The model under review builds one solid part; all positions refer to its coordinate system, in mm. A direction names the side the tool comes from. Coordinates: 2 decimals unless noted, no trailing zeros. Write each loop counter-clockwise with the first axis right and the second up, starting at its lowest first coordinate (ties: lowest second). Pieces come first, ordered by that corner, then holes.
```python
from build123d import *

# Parameters (mm, degrees)
SKETCH1_R               = 9.525
BOSS_EXTRUDE1_DEPTH     = 9.525
SKETCH2_R               = 3.175
BOSS_EXTRUDE2_DEPTH     = 12.7
SKETCH3_R               = 4.7625
CUT_EXTRUDE1_DEPTH      = 10.525
CUT_EXTRUDE1_DEPTH_BACK = 10.525


with BuildPart() as part:
    # Sketch1 → Boss-Extrude1 (new body, symmetric)
    with BuildSketch(Plane.XY):
        Circle(SKETCH1_R)
    extrude(amount=BOSS_EXTRUDE1_DEPTH, both=True)

    # Sketch2 → Boss-Extrude2 (add, symmetric)
    with BuildSketch(Plane.XY):
        Circle(SKETCH2_R)
    extrude(amount=BOSS_EXTRUDE2_DEPTH, both=True)

    # Sketch3 → Cut-Extrude1 (cut, two sides)
    with BuildSketch(Plane(origin=(0, 0, 0), x_dir=(0, 0, -1), z_dir=(1, 0, 0))) as cut_extrude1_sk:
        Circle(SKETCH3_R)
    extrude(amount=CUT_EXTRUDE1_DEPTH, mode=Mode.SUBTRACT)
    extrude(cut_extrude1_sk.sketch, amount=-CUT_EXTRUDE1_DEPTH_BACK, mode=Mode.SUBTRACT)


solid = part.part
```
Item 1: Take a section at D-D, the plane y = 2.5. Write out the cut boundary in (x, z) (3 decimals), plus the area to 3 significant figures.
Solved:
outline: (-9.191, -9.525) - (-1.957, -9.525) - (-1.957, -12.7) - (1.957, -12.7) - (1.957, -9.525) - (9.191, -9.525) - (9.191, -4.054) - (-9.191, -4.054) - close; (-9.191, 4.054) - (9.191, 4.054) - (9.191, 9.525) - (1.957, 9.525) - (1.957, 12.7) - (-1.957, 12.7) - (-1.957, 9.525) - (-9.191, 9.525) - close
area: 226 mm2
Item 2: Take a section at C-C, the plane z = 2.25. Write out the cut boundary in (x, y) (3 decimals).
Solved:
outline: (-8.55, -4.197) arc R9.525 ccw to (8.55, -4.197) - close; (-8.55, 4.197) - (8.55, 4.197) arc R9.525 ccw to start
Item 3: Take a section at A-A, the plane y = 0. Write out the cut boundary in (x, z) (1 decimal).
Solved:
outline: (-9.5, -9.5) - (-3.2, -9.5) - (-3.2, -12.7) - (3.2, -12.7) - (3.2, -9.5) - (9.5, -9.5) - (9.5, -4.8) - (-9.5, -4.8) - close; (-9.5, 4.8) - (9.5, 4.8) - (9.5, 9.5) - (3.2, 9.5) - (3.2, 12.7) - (-3.2, 12.7) - (-3.2, 9.5) - (-9.5, 9.5) - close
Item 4: Machinability: for faces 1 (the face through (-0.69, -3.1, 11.13)), 2 (the face through (0, 0, 12.7)), 3 (the face through (4, 0, -9.525)), which of the approach directions +Z, -Z, +X, -X, +Y, -Y give a long, thin tool a straight path to every point of the face, cutting with its end or side? Answer none if there is none.
Solved:
face 1: +Z
face 2: +Z, +X, -X, +Y, -Y
face 3: -Z
Item 5: To check wall thickness, follow line 1 along Z through (x, y) = (-2.5, 0); line 2 along Z through (x, y) = (4.75, 0) (1 decimal); line 3 along Y through (x, z) = (-5, 0). State the ranges of each line that lie inside material, in increasing order.
Solved:
line 1: z = -12.7 to -4.76, 4.76 to 12.7
line 2: z = -9.5 to -4.8, 4.8 to 9.5
line 3: y = -8.11 to -4.76, 4.76 to 8.11
Item 6: Take a section at B-B, the plane x = -3.5. Write out the cut boundary in (y, z) (1 decimal).
Solved:
outline: (-8.9, -9.5) - (8.9, -9.5) - (8.9, 9.5) - (-8.9, 9.5) - close; hole circle Ø9.5 at (0, 0)
Item 7: Mouldability with a two-part tool opening along Z and no side actions: class faces 4 (the face through (0, 0, -12.7)), 5 (the face through (4, 0, 9.525)), 6 (the face through (-0.69, -3.1, -11.09)) as pulls with the +Z half, pulls with the -Z half, needs draft (parallel to the pull), parting line crosses it, or undercut.
Solved:
face 4: pulls with the -Z half
face 5: pulls with the +Z half
face 6: needs draft
Item 8: For pin 1 (5 mm diameter, centred on y = -5, z = -9.5, fed in from +X); pin 2 (1 mm diameter, centred on y = -2.5, z = -8.5, fed in from -X); pin 3 (1.5 mm diameter, centred on x = -3, z = 7.5, fed in from +Y), all flat-tipped, find the tip position at first contact; note any pin that passes through.
Solved:
pin 1: stops at x = 9.19
pin 2: stops at x = -9.31
pin 3: stops at y = 9.26
